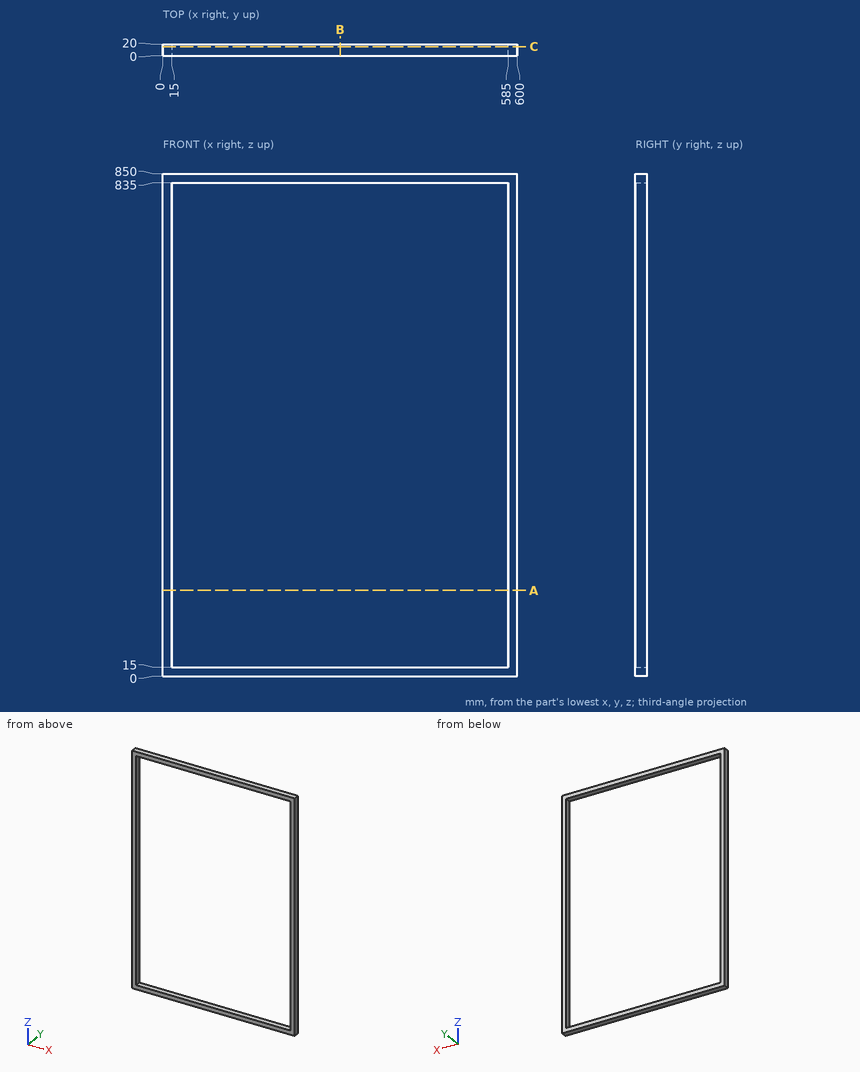
Answer from the drawing. Dimensions are ordinates in mm from the lowest x, y and z of the part. Round coordinates to 2 decimals unless told otherwise and drop trailing zeros. Loops run counter-clockwise (first coordinate to the right, second up) from the corner with the lowest first, then second, coordinate; pieces in that order, holes last.
(1) Find the intervals of material crossed by L1, parallel to Z at x = 440.5, y = 9; L2, parallel to X at y = 4.5, z = 464, in increasing order.
Computed values:
L1: z = 0 to 15, 835 to 850
L2: x = 0 to 15, 585 to 600
(2) The part is cut by section A-A, the plane z = 145. Give the vertices of the cut face in (x, y).
Computed values:
outline: (0, 0) - (15, 0) - (15, 20) - (0, 20) - close; (585, 0) - (600, 0) - (600, 20) - (585, 20) - close
(3) The part is cut by section C-C, the plane y = 15.5. Give the vertices of the cut face in (x, z).
Computed values:
outline: (0, 0) - (600, 0) - (600, 850) - (0, 850) - close; hole (15, 15) - (585, 15) - (585, 835) - (15, 835) - close
(4) The part is cut by section B-B, the plane x = 300. Give the vertices of the cut face in (y, z), and give its area (3 significant figures).
Computed values:
outline: (0, 0) - (20, 0) - (20, 15) - (0, 15) - close; (0, 835) - (20, 835) - (20, 850) - (0, 850) - close
area: 600 mm2
